Geometry: final body of the model. Coordinates: model frame, mm. Give positions to 0.01 mm unless a question says otherwise; leave off trailing zeros. Loops run counter-clockwise (first coordinate to the right, second up) from the corner with the lowest first, then second, coordinate; pieces in that order, holes last. Notation, with made-up numbers: (18, 82) -> (32, 82) arc R27 cw to (32, 106) -> close; hole circle Ø7 at (14, 69). An arc over 180 degrees is marked (long way). Answer in a Markdown table with one row per item. Add a question column.
1) Section query C-C (x = 0.75). Give the number of separate pieces and of enclosed holes in the cut face, plus the area to 3 significant figures.
2) Line query: line 1 (Z direction, x = 0.6, y = 25); line 2 (Y direction, x = 0.95, z = -145) (3 decimals); line 3 (Y direction, x = 1.1, z = -155). Output: solid intervals per line, ascending. Write a range as from..to.
3) First-contact query: P1, Ø5.5, axis at y = 75.35, z = -155, coming from the +X side (3 decimals); P2, Ø4.5, axis at y = 85.35, z = 135, coming from the +X side (3 decimals). Flat tips, straight axial feed; report the tip coordinate or a pass-through.
4) Draft query along Y for faces 1 (the cylindrical face through (1.61, 28.89, 127.31)), 2 (the flat face through (0, 66, 2)). Return one class per face: +Y half, -Y half, draft (parallel to the pull), parting line (faces both ways), or undercut.
5) Section query B-B (z = 48). Return the cut outline in (x, y) (3 decimals).
6) Section query A-A (y = 49.5). Return the cut outline in (x, z) (3 decimals), plus the area to 3 significant figures.
```python
from build123d import *

# Parameters (mm, degrees)
BOSS_EXTRUDE1_DEPTH                             = 3.175
CSK_FOR_M3_FLAT_HEAD_MACHINE_SCREW1_D           = 3.4
CSK_FOR_M3_FLAT_HEAD_MACHINE_SCREW1_CSINK_D     = 6.3
CSK_FOR_M3_FLAT_HEAD_MACHINE_SCREW1_CSINK_ANGLE = 90
SKETCH4_R                                       = 5
CUT_EXTRUDE1_DEPTH                              = 4.175


with BuildPart() as part:
    # Sketch1 → Boss-Extrude1 (new body)
    with BuildSketch(Plane(origin=(0, 0, 0), x_dir=(0, 0, -1), z_dir=(1, 0, 0))):
        Polygon((160, 0), (160, 3.175), (160, 47.175), (160, 50.35), (160, 60.35), (160, 90.35), (-160, 90.35), (-160, 60.35), (-160, 50.35), (-160, 47.175), (-160, 3.175), (-160, 0), align=None)
    extrude(amount=BOSS_EXTRUDE1_DEPTH)

    # CSK for M3 Flat Head Machine Screw1 (through all)
    with Locations(Plane(origin=(3.175, 0, 0), x_dir=(0, 0, -1), z_dir=(1, 0, 0))):
        with Locations((-145, 8.175), (-135, 8.175), (-105, 8.175), (-145, 55.35), (-135, 55.35), (-105, 55.35), (-117.5, 30.175), (-136.25, 19.349682453), (-136.25, 41.000317547), (-145, 85.35), (-135, 85.35), (-105, 85.35), (-155, 65.35), (-155, 75.35)):
            csk_for_m3_flat_head_machine_screw1 = CounterSinkHole(CSK_FOR_M3_FLAT_HEAD_MACHINE_SCREW1_D / 2, CSK_FOR_M3_FLAT_HEAD_MACHINE_SCREW1_CSINK_D / 2, counter_sink_angle=CSK_FOR_M3_FLAT_HEAD_MACHINE_SCREW1_CSINK_ANGLE)

    # Mirror1: CSK for M3 Flat Head Machine Screw1 across plane
    add(csk_for_m3_flat_head_machine_screw1.mirror(Plane.XY), mode=Mode.SUBTRACT)

    # Sketch4 → Cut-Extrude1 (cut, through all)
    with BuildSketch(Plane(origin=(3.175, 0, 0), x_dir=(0, 0, -1), z_dir=(1, 0, 0))):
        with Locations((-130, 24.675)):
            Circle(SKETCH4_R)
        with Locations((130, 24.675)):
            Circle(SKETCH4_R)
        with BuildLine():
            Line((-100, 57.35), (-100, 0))
            Line((-100, 0), (100, 0))
            Line((100, 0), (100, 57.35))
            ThreePointArc((100, 57.35), (99.121320344, 59.471320344), (97, 60.35))
            Line((97, 60.35), (-97, 60.35))
            ThreePointArc((-97, 60.35), (-99.121320344, 59.471320344), (-100, 57.35))
        make_face()
    extrude(amount=-CUT_EXTRUDE1_DEPTH, mode=Mode.SUBTRACT)


solid = part.part
```
Evaluation:
| question | item | result |
|---|---|---|
| 1 | separate pieces | 1 |
| 1 | enclosed holes | 30 |
| 1 | area | 16,400 mm² |
| 2 | line 1 | -160..-134.99, -125.01..-100, 100..125.01, 134.99..160 |
| 2 | line 2 | 0..6.475, 9.875..53.65, 57.05..83.65, 87.05..90.35 |
| 2 | line 3 | 0..63.65, 67.05..73.65, 77.05..90.35 |
| 3 | P1 | x = 2.775 |
| 3 | P2 | x = 2.275 |
| 4 | face 1 | undercut |
| 4 | face 2 | draft |
| 5 | outline | (0, 60.35) -> (3.175, 60.35) -> (3.175, 90.35) -> (0, 90.35) -> close |
| 6 | outline | (0, -160) -> (3.175, -160) -> (3.175, -100) -> (0, -100) -> close; (0, 100) -> (3.175, 100) -> (3.175, 160) -> (0, 160) -> close |
| 6 | area | 381 mm² |
